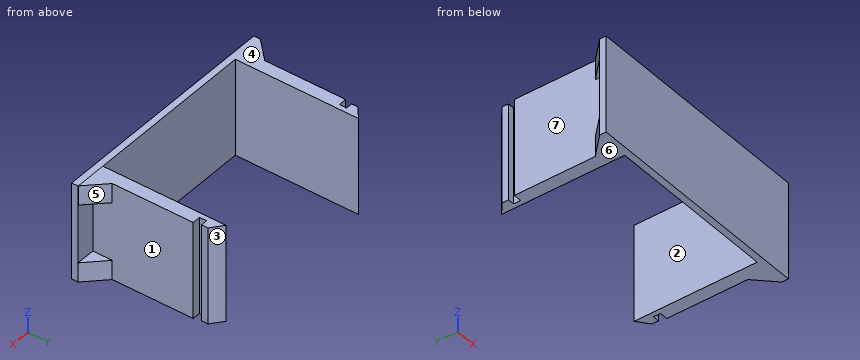
```python
from build123d import *

# Parameters (mm, degrees)
SKETCH2_W             = 4
SKETCH2_H             = 29.975509742
BOSS_EXTRUDE1_DEPTH   = 38
BOSS_EXTRUDE1_2_DEPTH = 38
SKETCH3_W             = 72.876339672
SKETCH3_H             = 29.975509742
BOSS_EXTRUDE3_DEPTH   = 2
BOSS_EXTRUDE4_DEPTH   = 6
BOSS_EXTRUDE5_DEPTH   = 6
BOSS_EXTRUDE7_DEPTH   = 6
BOSS_EXTRUDE8_DEPTH   = 6
SKETCH17_W            = 32.717324733
SKETCH17_H            = 7
CUT_EXTRUDE9_DEPTH    = 0.5
SKETCH18_W            = 40.099699831
SKETCH18_H            = 2.2
CUT_EXTRUDE10_DEPTH   = 2
CUT_EXTRUDE11_DEPTH   = 31
SKETCH20_W            = 49.216753152
SKETCH20_H            = 10.950019834
CUT_EXTRUDE12_DEPTH   = 0.5
SKETCH21_W            = 42.54396611
SKETCH21_H            = 2.2
CUT_EXTRUDE13_DEPTH   = 2
CUT_EXTRUDE14_DEPTH   = 30.975509742


with BuildPart() as part:
    # Sketch2 → Boss-Extrude1 (new body)
    with BuildSketch(Plane(origin=(0, 0, 0), x_dir=(1, 0, 0), z_dir=(0, 1, 0))):
        with Locations((-22.117643943, -3.05661445)):
            Rectangle(SKETCH2_W, SKETCH2_H)
    extrude(amount=BOSS_EXTRUDE1_DEPTH)



with BuildPart() as body_2:
    # Sketch2 → Boss-Extrude1 2 (new body)
    with BuildSketch(Plane(origin=(0, 0, 0), x_dir=(1, 0, 0), z_dir=(0, 1, 0))):
        Polygon((36.882356057, 11.931140421), (35.682356057, 11.931140421), (32.882356057, 11.931140421), (32.882356057, -18.068859579), (36.882356057, -18.068859579), align=None)
    extrude(amount=BOSS_EXTRUDE1_2_DEPTH)


with BuildPart() as part_1:
    add(part.part)

    add(body_2.part)  # Boss-Extrude3 merges body 2
    # Sketch3 → Boss-Extrude3 (add)
    with BuildSketch(Plane(origin=(0, 0, 0), x_dir=(1, 0, 0), z_dir=(0, 1, 0))):
        with Locations((6.320525893, -3.05661445)):
            Rectangle(SKETCH3_W, SKETCH3_H)
    extrude(amount=-BOSS_EXTRUDE3_DEPTH)

    # Sketch6 → Boss-Extrude4 (add)
    with BuildSketch(Plane.XY.offset(18.068859579)):
        Polygon((36.882356057, 6), (36.882356057, 0), (42.682356057, 0), align=None)
    extrude(amount=-BOSS_EXTRUDE4_DEPTH)

    # Sketch7 → Boss-Extrude5 (add)
    with BuildSketch(Plane(origin=(0, 0, -11.931140421), x_dir=(-1, 0, 0), z_dir=(0, 0, -1))):
        Polygon((-42.758695729, 0), (-36.882356057, 6), (-36.882356057, 0), align=None)
    extrude(amount=-BOSS_EXTRUDE5_DEPTH)

    # Sketch9 → Boss-Extrude7 (add)
    with BuildSketch(Plane.XY.offset(18.044369321)):
        Polygon((-24.117643943, 6), (-30.117643943, 0), (-24.117643943, 0), align=None)
    extrude(amount=-BOSS_EXTRUDE7_DEPTH)

    # Sketch8 → Boss-Extrude8 (add)
    with BuildSketch(Plane(origin=(0, 0, -11.931140421), x_dir=(-1, 0, 0), z_dir=(0, 0, -1))):
        Polygon((24.117643943, 6), (24.117643943, 0), (30.117643943, 0), align=None)
    extrude(amount=-BOSS_EXTRUDE8_DEPTH)

    # Sketch17 → Cut-Extrude9 (cut)
    with BuildSketch(Plane(origin=(36.882356057, 0, 0), x_dir=(0, 0, -1), z_dir=(1, 0, 0))):
        with Locations((-4.427521945, 34.5)):
            Rectangle(SKETCH17_W, SKETCH17_H)
    extrude(amount=-CUT_EXTRUDE9_DEPTH, mode=Mode.SUBTRACT)

    # Sketch18 → Cut-Extrude10 (cut)
    with BuildSketch(Plane(origin=(36.382356057, 0, 0), x_dir=(0, 0, -1), z_dir=(1, 0, 0))):
        with Locations((1.980990336, 32.1)):
            Rectangle(SKETCH18_W, SKETCH18_H)
    extrude(amount=-CUT_EXTRUDE10_DEPTH, mode=Mode.SUBTRACT)

    # Sketch19 → Cut-Extrude11 (cut, through all)
    with BuildSketch(Plane.XY.offset(18.068859579)):
        Polygon((36.382356057, 35.2), (32.882356057, 38), (30.81845706, 44.907759877), (43.465809669, 41.162121973), align=None)
    extrude(amount=-CUT_EXTRUDE11_DEPTH, mode=Mode.SUBTRACT)

    # Sketch20 → Cut-Extrude12 (cut)
    with BuildSketch(Plane.ZY.offset(24.117643943)):
        with Locations((-6.564007255, 36.475009917)):
            Rectangle(SKETCH20_W, SKETCH20_H)
    extrude(amount=-CUT_EXTRUDE12_DEPTH, mode=Mode.SUBTRACT)

    # Sketch21 → Cut-Extrude13 (cut)
    with BuildSketch(Plane.ZY.offset(23.617643943)):
        with Locations((-3.227613734, 32.1)):
            Rectangle(SKETCH21_W, SKETCH21_H)
    extrude(amount=-CUT_EXTRUDE13_DEPTH, mode=Mode.SUBTRACT)

    # Sketch22 → Cut-Extrude14 (cut, through all)
    with BuildSketch(Plane.XY.offset(18.044369321)):
        Polygon((-23.617643943, 35.2), (-20.117643943, 38), (-17.308564487, 46.700014394), (-43.949503764, 46.700014394), (-33.84948937, 36.6), align=None)
    extrude(amount=-CUT_EXTRUDE14_DEPTH, mode=Mode.SUBTRACT)


solid = part_1.part
```
Can you work these out from the model? Positions are in its coordinate system, mm. Face numbers are marked on the shaded views. A direction names the side the tool comes from. Coordinates: 2 decimals unless noted, no trailing zeros. Write each loop counter-clockwise with the first axis right and the second up, starting at its lowest first coordinate (ties: lowest second). Pieces come first, ordered by that corner, then holes. Notation, with made-up numbers: M 20.5,-10.75 L 76.5,-10.75 A18 cw 76.5,24.25 Z; hole C 75,-11.75 d9. An arc over 180 degrees is marked long. Answer as CSV lines item,"result".
Item 1: Please list where these lines run through material, in increasing order: line 1 along X through (y, z) = (7, 0); line 2 along X through (y, z) = (34, -3); line 3 along Y through (x, z) = (27, 16.5).
Geometry results:
line 1,"x = -24.12 to -20.12, 32.88 to 36.88"
line 2,"x = -23.62 to -20.12, 32.88 to 36.38"
line 3,"y = -2 to 0"
Item 2: Imagine slicing it at C-C on y = 32. List the corners of the cut face in (x, z) for me.
Geometry results:
outline,"M -21.62,-11.93 L -20.12,-11.93 L -20.12,18.04 L -21.62,18.04 Z; M 32.88,-11.93 L 34.38,-11.93 L 34.38,18.07 L 32.88,18.07 Z"
Item 3: Imagine slicing it at B-B on z = 10.5. List the corners of the cut face in (x, y) for me, plus the area to 3 significant figures.
Geometry results:
outline,"M -30.12,-2 L 42.76,-2 L 42.76,0 L 36.88,0 L 36.88,31 L 34.38,31 L 34.38,33.2 L 36.38,33.2 L 36.38,35.2 L 32.88,38 L 32.88,0 L -20.12,0 L -20.12,38 L -23.62,35.2 L -23.62,33.2 L -21.62,33.2 L -21.62,31 L -24.12,31 L -24.12,0 L -30.12,0 Z"
area,"424 mm2"
Item 4: Imagine slicing it at D-D on z = 16.5. List the corners of the cut face in (x, y) for me.
Geometry results:
outline,"M -30.12,-2 L 42.76,-2 L 42.76,0 L 42.68,0 L 36.88,6 L 36.88,31 L 34.38,31 L 34.38,33.2 L 36.38,33.2 L 36.38,35.2 L 32.88,38 L 32.88,0 L -20.12,0 L -20.12,38 L -23.62,35.2 L -23.62,33.2 L -21.62,33.2 L -21.62,31 L -24.12,31 L -24.12,6 L -30.12,0 Z"
Item 5: I'm going to push flat-ended pins straight in: P1, Ø8, axis at y = 15, z = 13.5, coming from the -X side; P2, Ø9, axis at x = 3.5, z = 0, coming from the +Y side; P3, Ø1.2, axis at x = -22.5, z = -0.5, coming from the +Y side. Where does each tip first touch, or does it pass through?
Geometry results:
P1,"stops at x = -24.12"
P2,"stops at y = 0"
P3,"stops at y = 36.57"
Item 6: We'd pull the mould along Z, two halves only. Please class the marked faces 4, 5, 6 and 7: +Z half, -Z half, draft (parallel to the pull), parting line (faces both ways), or undercut.
Geometry results:
face 4,"+Z half"
face 5,"draft"
face 6,"-Z half"
face 7,"undercut"
Item 7: Imagine slicing it at A-A on y = 23. List the corners of the cut face in (x, z) for me, plus the area to 3 significant figures.
Geometry results:
outline,"M -24.12,-11.93 L -20.12,-11.93 L -20.12,18.04 L -24.12,18.04 Z; M 32.88,-11.93 L 36.88,-11.93 L 36.88,18.07 L 32.88,18.07 Z"
area,"240 mm2"
Item 8: On a 3-axis mill with a long thin cutter (end or side, diameter ignored), from which of +Z, -Z, +X, -X, +Y, -Y can I reach the whole of each face in a straight line? I mean the marked faces 1, 2 and 3. Say none if no direction works.
Geometry results:
face 1,"+X, +Y"
face 2,"+Z, -Z, +Y"
face 3,"+Z, -Z, +X, +Y"
